from build123d import *

# Parameters (mm, degrees)
SKETCH1_W           = 100
SKETCH1_H           = 18
SKETCH1_W_2         = 5
SKETCH1_H_2         = 7
SKETCH1_W_3         = 3.5
SKETCH1_H_3         = 6
SKETCH1_H_4         = 6.5
BOSS_EXTRUDE1_DEPTH = 1
SKETCH2_W           = 3.5
SKETCH2_H           = 6
BOSS_EXTRUDE2_DEPTH = 3.5
BOSS_EXTRUDE2_TAPER = -20
SKETCH3_W           = 6.04779164
SKETCH3_H           = 1.5
CUT_EXTRUDE1_DEPTH  = 2.5
SKETCH4_W           = 3.5
SKETCH4_H           = 6.5
BOSS_EXTRUDE3_DEPTH = 3
BOSS_EXTRUDE4_DEPTH = 6.5
SKETCH10_R          = 1.8
SKETCH10_R_2        = 1.85
SKETCH10_R_3        = 1.9
SKETCH10_R_4        = 1.95
SKETCH10_R_5        = 2
CUT_EXTRUDE2_DEPTH  = 2
SKETCH10_3_R        = 1.45
SKETCH10_3_R_2      = 1.5
SKETCH10_3_R_3      = 1.55
SKETCH10_3_R_4      = 1.6
SKETCH10_3_R_5      = 1.65
BOSS_EXTRUDE5_DEPTH = 2
BOSS_EXTRUDE5_TAPER = -10


with BuildPart() as part:
    # Sketch1 → Boss-Extrude1 (new body)
    with BuildSketch(Plane(origin=(0, 0, 0), x_dir=(1, 0, 0), z_dir=(0, 1, 0))):
        with Locations((50, 9)):
            Rectangle(SKETCH1_W, SKETCH1_H)
        with Locations((7.5, 9)):
            Rectangle(SKETCH1_W_2, SKETCH1_H_2, mode=Mode.SUBTRACT)
        with Locations((93.25, 9)):
            Rectangle(SKETCH1_W_3, SKETCH1_H_3, mode=Mode.SUBTRACT)
        with Locations((19.340066027, 9)):
            Rectangle(SKETCH1_W_3, SKETCH1_H_4, mode=Mode.SUBTRACT)
    extrude(amount=BOSS_EXTRUDE1_DEPTH)

    # Sketch2 → Boss-Extrude2 (add)
    with BuildSketch(Plane.XZ):
        with Locations((93.25, -9)):
            Rectangle(SKETCH2_W, SKETCH2_H)
    extrude(amount=-BOSS_EXTRUDE2_DEPTH, taper=BOSS_EXTRUDE2_TAPER)

    # Sketch3 → Cut-Extrude1 (cut)
    with BuildSketch(Plane(origin=(0, 3.5, 0), x_dir=(1, 0, 0), z_dir=(0, 1, 0))):
        with Locations((93.25, 9)):
            Rectangle(SKETCH3_W, SKETCH3_H)
    extrude(amount=-CUT_EXTRUDE1_DEPTH, mode=Mode.SUBTRACT)

    # Sketch4 → Boss-Extrude3 (add)
    with BuildSketch(Plane.XZ):
        with Locations((19.340066027, -9)):
            Rectangle(SKETCH4_W, SKETCH4_H)
    extrude(amount=-BOSS_EXTRUDE3_DEPTH)

    # Sketch9 → Boss-Extrude4 (add)
    with BuildSketch(Plane(origin=(0, 0, -12.25), x_dir=(-1, 0, 0), z_dir=(0, 0, -1))):
        Polygon((-31.411175368, 3), (-27.911175368, 3), (-27.038919355, 0), (-30.538919355, 0), align=None)
    extrude(amount=-BOSS_EXTRUDE4_DEPTH)

    # Sketch10 → Cut-Extrude2 (cut, through all)
    with BuildSketch(Plane(origin=(0, 1, 0), x_dir=(1, 0, 0), z_dir=(0, 1, 0))):
        with Locations((83.971192641, 5.901209197)):
            Circle(SKETCH10_R)
        with Locations((75.205441642, 5.901209197)):
            Circle(SKETCH10_R_2)
        with Locations((65.048301596, 5.901209197)):
            Circle(SKETCH10_R_3)
        with Locations((55.169439359, 5.901209197)):
            Circle(SKETCH10_R_4)
        with Locations((44.873160409, 5.901209197)):
            Circle(SKETCH10_R_5)
    extrude(amount=-CUT_EXTRUDE2_DEPTH, mode=Mode.SUBTRACT)

    # Sketch10<3> → Boss-Extrude5 (add)
    with BuildSketch(Plane(origin=(0, 1, 0), x_dir=(1, 0, 0), z_dir=(0, 1, 0))):
        with Locations((79.727456046, 11.814612648)):
            Circle(SKETCH10_3_R)
        with Locations((69.918163262, 11.814612648)):
            Circle(SKETCH10_3_R_2)
        with Locations((60.108870478, 11.814612648)):
            Circle(SKETCH10_3_R_3)
        with Locations((49.812591527, 11.814612648)):
            Circle(SKETCH10_3_R_4)
        with Locations((40.142437647, 11.814612648)):
            Circle(SKETCH10_3_R_5)
    extrude(amount=BOSS_EXTRUDE5_DEPTH, taper=BOSS_EXTRUDE5_TAPER)


solid = part.part
Model file for the job. Use its own axes, mm. A direction names the side the tool comes from. Give positions to 0.01 mm unless a question says otherwise; leave off trailing zeros. Write each loop counter-clockwise with the first axis right and the second up, starting at its lowest first coordinate (ties: lowest second). Pieces come first, ordered by that corner, then holes. Notation, with made-up numbers: M 89,67.25 L 132,67.25 A15 ccw 132,75.25 Z; hole C -24,26.5 d2. An arc over 180 degrees is marked long. One line per item, written item: value. Start each with the question number.
Q1. Probe probe 1 along X at (y, z) = (2.4, -12.75); probe 2 along X at (y, z) = (0.5, -8.25); probe 3 along X at (y, z) = (1.15, -13). List the from-to ranges inside material, lowest first. Write a range as [from, to].
Q2. 3-axis set-ups, long thin cutter, end or side, ignore diameter. For faces 4 (the flat face through (70, 3, -12)), 5 (the flat face through (29, 2, -12.25)), 6 (the flat face through (27.624, 2.014, -9.046)): which of +Z, -Z, +X, -X, +Y, -Y reach the whole face in a straight line?
Q3. Drop flat-ended pins along their axis: pin 1 Ø1.2 at (x, z) = (49.5, -12.5) entering from +Y; pin 2 Ø1.3 at (x, y) = (94.5, 2.5) entering from +Z; pin 3 Ø1.6 at (x, y) = (29, 2) entering from +Z; pin 4 Ø1.1 at (x, y) = (8, 0.5) entering from +Z. Give the stop position or say it passes through.
Q4. Saw through at B-B, the plane z = -1.5. Write the cut outline in (x, y).
Q5. Saw through at A-A, the plane x = 76. Write the cut outline in (y, z).
Q6. Saw through at C-C, the plane y = 1.7. State how many separate pieces and enclosed holes the cut face has, plus the area to 3 significant figures.
Q7. Two-plate mould, pull along Z, no slides. Class faces 1 (the cylindrical face through (56.97, 0.51, -5.15)), 2 (the flat face through (29, 2, -5.75)), 3 (the flat face through (21.09, 2, -9)): +Z half, -Z half, draft (parallel to the pull), parting line (faces both ways), or undercut.
Output values:
1. probe 1: x = [38.49, 41.79], [48.22, 51.41], [58.57, 61.64], [68.44, 71.39], [78.31, 81.14], [90.63, 95.87]
1. probe 2: x = [0, 5], [10, 100]
1. probe 3: x = [38.96, 41.33], [48.7, 50.93], [59.07, 61.15], [68.96, 70.88], [78.85, 80.61]
2. face 4: +Z, -Z, -X, +Y
2. face 5: -Z, -X, +Y
2. face 6: +Z, -Z, +Y
3. pin 1: stops at y = 3
3. pin 2: stops at z = -4.85
3. pin 3: stops at z = -5.75
3. pin 4: stops at z = 0
4. outline: M 0,0 L 100,0 L 100,1 L 0,1 Z
5. outline: M 0,-18 L 1,-18 L 1,-7.57 L 0,-7.57 Z; M 0,-4.23 L 1,-4.23 L 1,0 L 0,0 Z
6. separate pieces: 9
6. enclosed holes: 0
6. area: 117 mm²
7. face 1: undercut
7. face 2: +Z half
7. face 3: draft
